Geometry: see drawing. Coordinates: mm, zero at the bounding-box minimum. A direction names the side the tool comes from. Give positions to 0.01 mm unless a question says otherwise; leave off trailing zeros. Write each loop counter-clockwise with the first axis right and the second up, starting at its lowest first coordinate (ties: lowest second). Pieces come first, ordered by that corner, then holes.
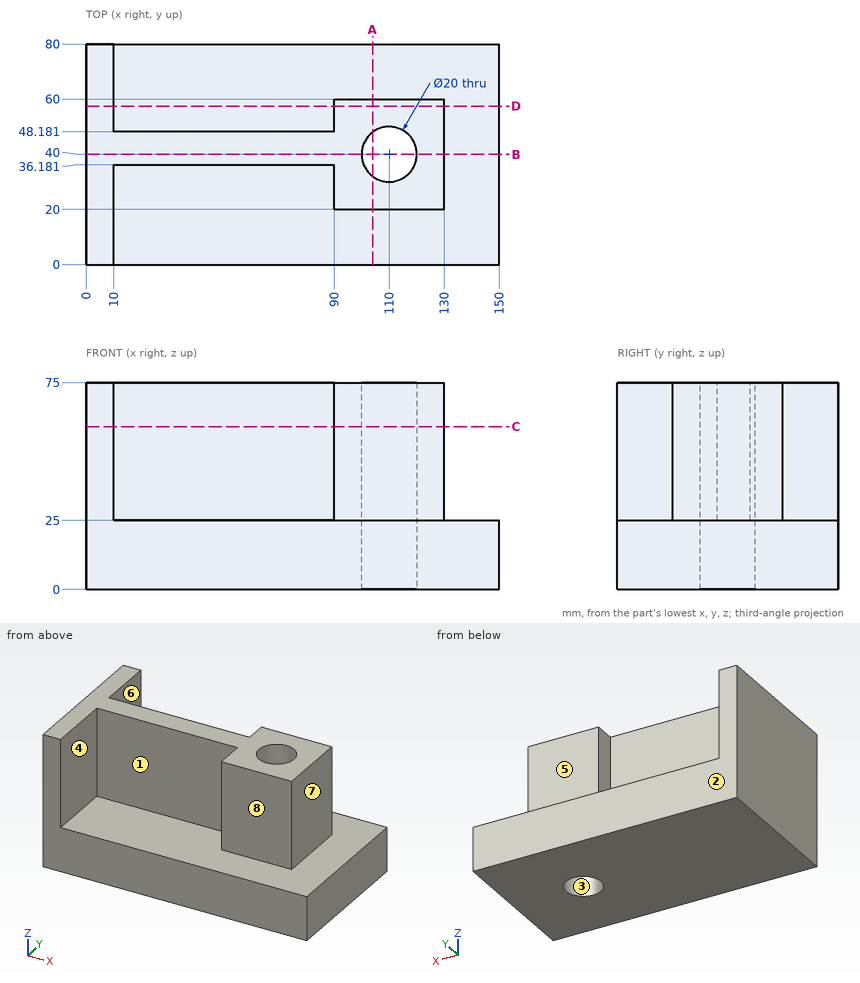
Q1. Pin query (flat end, axial travel): pin 1 (3 mm diameter, centred on x = 135, y = 32.5, fed in from -Z); pin 2 (9.5 mm diameter, centred on y = 58, z = 60.5, fed in from +X); pin 3 (20 mm diameter, centred on x = 103, z = 44.5, fed in from +Y); pin 4 (2 mm diameter, centred on x = 118.5, z = 51.5, fed in from -Y). Return the tip coordinate at first contact, or that it passes through.
Q2. Material intervals for line 1 along Y through (x, z) = (110, 48); line 2 along Y through (x, z) = (110, 24.5); line 3 along Z through (x, y) = (84, 65), sorted ascending.
Q3. Section D-D, the plane y = 57.5. Return the cut outline in (x, z).
Q4. Mould query, pull axis Y, two halves, no side actions, for the marked faces 1, 2 and 3. Classes: +Y half, -Y half, draft (parallel to the pull), parting line (faces both ways), or undercut.
Q5. Access query for the marked faces 4, 5, 6, 7 and 8. Directions: +Z, -Z, +X, -X, +Y, -Y. A direction counts if a zero-diameter tool reaches every point of the face in a straight line with its end or side. Return the directions, or none.
Q6. Section B-B, the plane y = 40. Return the cut outline in (x, z), then the cut area to 3 significant figures.
Q7. Section A-A, the plane x = 104. Return the cut outline in (y, z), then the cut area to 3 significant figures.
Q8. Section C-C, the plane z = 59. Return the cut outline in (x, y).
Solutions:
1. pin 1: stops at z = 0
1. pin 2: stops at x = 130
1. pin 3: stops at y = 60
1. pin 4: stops at y = 20
2. line 1: y = 20 to 30, 50 to 60
2. line 2: y = 0 to 30, 50 to 80
2. line 3: z = 0 to 25
3. outline: (0, 0) - (150, 0) - (150, 25) - (130, 25) - (130, 75) - (90, 75) - (90, 25) - (10, 25) - (10, 75) - (0, 75) - close
4. face 1: -Y half
4. face 2: +Y half
4. face 3: undercut
5. face 4: +Z, -Y
5. face 5: +Z, +X, +Y
5. face 6: +Z, +Y
5. face 7: +Z, +X, +Y, -Y
5. face 8: +Z, +X, -Y
6. outline: (0, 0) - (100, 0) - (100, 75) - (0, 75) - close; (120, 0) - (150, 0) - (150, 25) - (130, 25) - (130, 75) - (120, 75) - close
6. area: 8,750 mm2
7. outline: (0, 0) - (32, 0) - (32, 75) - (20, 75) - (20, 25) - (0, 25) - close; (48, 0) - (80, 0) - (80, 25) - (60, 25) - (60, 75) - (48, 75) - close
7. area: 2,800 mm2
8. outline: (0, 0) - (10, 0) - (10, 36.18) - (90, 36.18) - (90, 20) - (130, 20) - (130, 60) - (90, 60) - (90, 48.18) - (10, 48.18) - (10, 80) - (0, 80) - close; hole circle Ø20 at (110, 40)
